Could you check a few things on this drawing? It's one solid part, dimensions in mm from its lowest x, y, z. Round coordinates to 2 decimals unless told otherwise and drop trailing zeros. Write each loop counter-clockwise with the first axis right and the second up, starting at its lowest first coordinate (ties: lowest second). Pieces come first, ordered by that corner, then holes. Notation, with made-up numbers: (43, 16) -> (47, 16) arc R16 ccw to (47, 46) -> close; hole circle Ø3 at (-27, 84.25). An arc over 180 degrees is marked (long way). Answer in a Markdown table with one row per item.
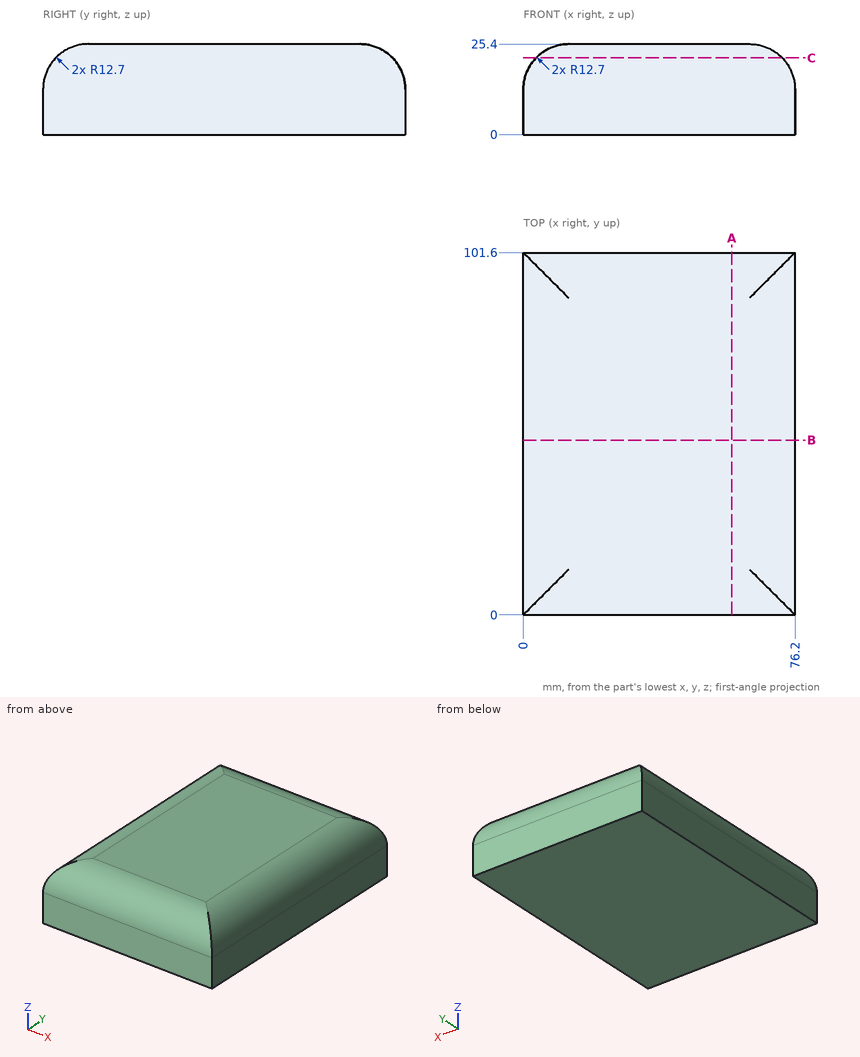
1) For pin 1 (12 mm diameter, centred on x = 11, z = 20.5, fed in from -Y); pin 2 (8 mm diameter, centred on x = 63, z = 17, fed in from -Y); pin 3 (4 mm diameter, centred on y = 18.5, z = 21.5, fed in from +X), each with a flat end and sliding along its axis, tell me the tip position at first contact or that it passes through.
Response:
| item | result |
|---|---|
| pin 1 | stops at y = 0.13 |
| pin 2 | stops at y = 0 |
| pin 3 | stops at x = 74.23 |
2) I want a section at C-C, the plane z = 21.5. List the corners of the cut face in (x, y) for me, and give its area (3 significant figures).
Response:
| item | result |
|---|---|
| outline | (3.54, 3.54) -> (72.66, 3.54) -> (72.66, 98.06) -> (3.54, 98.06) -> close |
| area | 6,530 mm^2 |
3) I want a section at A-A, the plane x = 58.5. List the corners of the cut face in (y, z) for me.
Response:
| item | result |
|---|---|
| outline | (0, 0) -> (101.6, 0) -> (101.6, 12.7) arc R12.7 ccw to (88.9, 25.4) -> (12.7, 25.4) arc R12.7 ccw to (0, 12.7) -> close |
4) I need wall thicknesses on line 1 (Z direction, x = 12.5, y = 31.5); line 2 (Y direction, x = 59, z = 13); line 3 (X direction, y = 31, z = 21.25). Which ranges of each line are inside material? Lowest first, please. Write a range as [from, to].
Response:
| item | result |
|---|---|
| line 1 | z = [0, 25.4] |
| line 2 | y = [0, 101.6] |
| line 3 | x = [3.31, 72.89] |
5) I want a section at B-B, the plane y = 49. List the corners of the cut face in (x, z) for me.
Response:
| item | result |
|---|---|
| outline | (0, 0) -> (76.2, 0) -> (76.2, 12.7) arc R12.7 ccw to (63.5, 25.4) -> (12.7, 25.4) arc R12.7 ccw to (0, 12.7) -> close |
